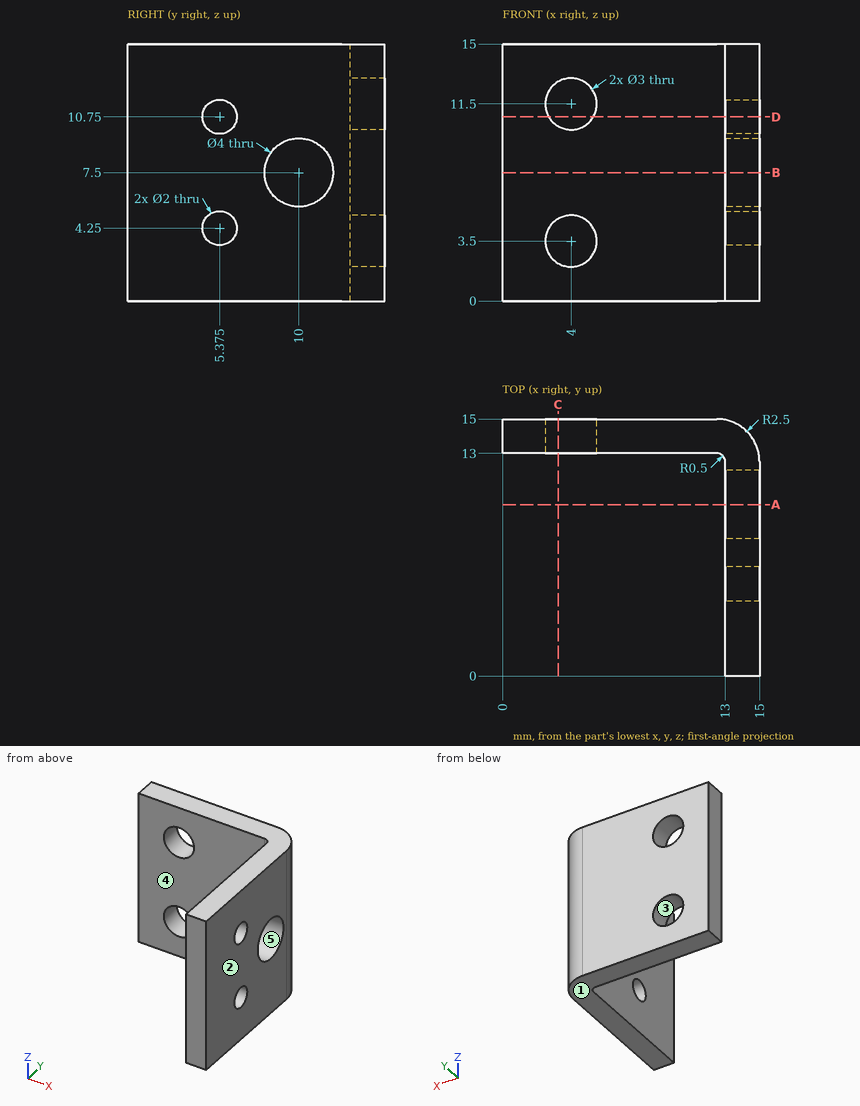
Design review of the part shown in the three views and the two pictorial views. Dimensions are in mm from the part's minimum x, y and z. A direction names the side the tool comes from. Round coordinates to 2 decimals unless told otherwise and drop trailing zeros. Write each loop counter-clockwise with the first axis right and the second up, starting at its lowest first coordinate (ties: lowest second). Pieces come first, ordered by that corner, then holes.
1) Take a section at B-B on z = 7.5. Give the boundary of the cut face in (x, y).
Answer below:
outline: (0, 13) - (12.5, 13) arc R0.5 cw to (13, 12.5) - (13, 12) - (15, 12) - (15, 12.5) arc R2.5 ccw to (12.5, 15) - (0, 15) - close; (13, 0) - (15, 0) - (15, 8) - (13, 8) - close
2) Take a section at D-D on z = 10.75. Give the boundary of the cut face in (x, y) (3 decimals), then the cut area to 3 significant figures.
Answer below:
outline: (0, 13) - (2.701, 13) - (2.701, 15) - (0, 15) - close; (5.299, 13) - (12.5, 13) arc R0.5 cw to (13, 12.5) - (13, 6.375) - (15, 6.375) - (15, 12.5) arc R2.5 ccw to (12.5, 15) - (5.299, 15) - close; (13, 0) - (15, 0) - (15, 4.375) - (13, 4.375) - close
area: 45.5 mm2
3) Mouldability with a two-part tool opening along X and no side actions: class the marked faces 1, 2 and 3 as +X half, -X half, draft (parallel to the pull), parting line (faces both ways), or undercut.
Answer below:
face 1: draft
face 2: +X half
face 3: undercut
4) Take a section at C-C on x = 3.25. Give the boundary of the cut face in (y, z), then the cut area to 3 significant figures.
Answer below:
outline: (13, 0) - (15, 0) - (15, 2.2) - (13, 2.2) - close; (13, 4.8) - (15, 4.8) - (15, 10.2) - (13, 10.2) - close; (13, 12.8) - (15, 12.8) - (15, 15) - (13, 15) - close
area: 19.6 mm2
5) Insertion check: pin 1 Ø4 at (x, z) = (4, 3.5) entering from -Y; pin 2 Ø3 at (y, z) = (10, 7.5) entering from +X; pin 3 Ø2.5 at (y, z) = (5.375, 10.75) entering from -X. Each pin has a flat end and moves straight along its axis. Give the tip position at first contact, or say it passes through.
Answer below:
pin 1: stops at y = 13
pin 2: passes through
pin 3: stops at x = 13
6) For line 1 along Z through (x, y) = (4, 13.65); line 2 along X through (y, z) = (9, 2.5), list the stretches that pass through material, from the lowest coordinate up.
Answer below:
line 1: z = 0 to 2, 5 to 10, 13 to 15
line 2: x = 13 to 15
7) Machinability: for the marked faces 4 and 5, which of the approach directions +Z, -Z, +X, -X, +Y, -Y give a long, thin tool a straight path to every point of the face, cutting with its end or side? Answer none if there is none.
Answer below:
face 4: +Z, -Z, -X, -Y
face 5: +X, -X
8) Take a section at A-A on y = 10. Give the boundary of the cut face in (x, z).
Answer below:
outline: (13, 0) - (15, 0) - (15, 5.5) - (13, 5.5) - close; (13, 9.5) - (15, 9.5) - (15, 15) - (13, 15) - close
